Model file for the job. Use its own axes, mm. Face numbers are marked on the shaded views. A direction names the side the tool comes from. Coordinates: 2 decimals unless noted, no trailing zeros. Order: outer loops, then holes, each group sorted by start corner. A loop starts at its lowest first (then second) coordinate and runs counter-clockwise, first axis right, second up.
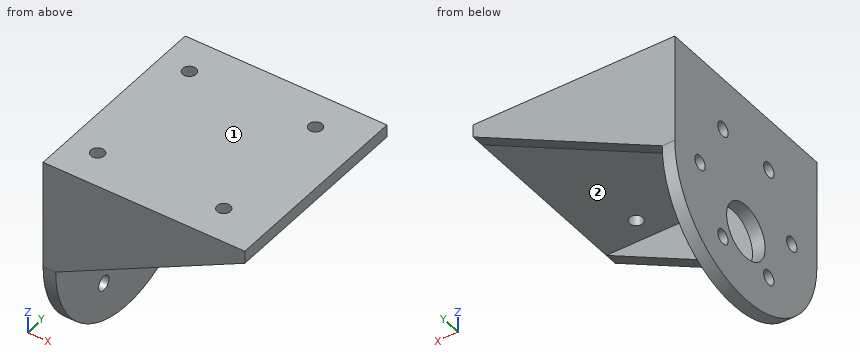
from build123d import *

# Parameters (mm, degrees)
SKETCH1_W           = 45
SKETCH1_H           = 48
SKETCH1_R           = 1.6
BOSS_EXTRUDE1_DEPTH = 3
BOSS_EXTRUDE2_DEPTH = 3
SKETCH4_R           = 6.5
SKETCH4_R_2         = 1.75
CUT_EXTRUDE1_DEPTH  = 10
BOSS_EXTRUDE3_DEPTH = 3
BOSS_EXTRUDE4_START = -48
BOSS_EXTRUDE4_DEPTH = 3


with BuildPart() as part:
    # Sketch1 → Boss-Extrude1 (new body)
    with BuildSketch(Plane.XY):
        with Locations((22.5, 24)):
            Rectangle(SKETCH1_W, SKETCH1_H)
        with Locations((4, 8.5)):
            Circle(SKETCH1_R, mode=Mode.SUBTRACT)
        with Locations((4, 39.5)):
            Circle(SKETCH1_R, mode=Mode.SUBTRACT)
        with Locations((34, 8.5)):
            Circle(SKETCH1_R, mode=Mode.SUBTRACT)
        with Locations((34, 39.5)):
            Circle(SKETCH1_R, mode=Mode.SUBTRACT)
    extrude(amount=BOSS_EXTRUDE1_DEPTH)

    # Sketch2 → Boss-Extrude2 (add)
    with BuildSketch(Plane.ZY):
        with BuildLine():
            Line((3, 48), (-23, 48))
            ThreePointArc((-23, 48), (-47, 24), (-23, 0))
            Line((-23, 0), (3, 0))
            Line((3, 0), (3, 48))
        make_face()
    extrude(amount=BOSS_EXTRUDE2_DEPTH)

    # Sketch4 → Cut-Extrude1 (cut)
    with BuildSketch(Plane.ZY.offset(3)):
        with Locations((-30, 24)):
            Circle(SKETCH4_R)
        with Locations((-23, 39.5)):
            Circle(SKETCH4_R_2)
        with Locations((-9.576606241, 31.75)):
            Circle(SKETCH4_R_2)
        with Locations((-9.576606241, 16.25)):
            Circle(SKETCH4_R_2)
        with Locations((-23, 8.5)):
            Circle(SKETCH4_R_2)
        with Locations((-36.423393759, 16.25)):
            Circle(SKETCH4_R_2)
        with Locations((-36.423393759, 31.75)):
            Circle(SKETCH4_R_2)
    extrude(amount=-CUT_EXTRUDE1_DEPTH, mode=Mode.SUBTRACT)

    # Sketch5 → Boss-Extrude3 (add)
    with BuildSketch(Plane(origin=(0, 48, 0), x_dir=(1, 0, 0), z_dir=(0, 1, 0))):
        Polygon((0, 23), (45, 0), (0, 0), align=None)
    extrude(amount=-BOSS_EXTRUDE3_DEPTH)

    # Sketch5<2> → Boss-Extrude4 (add)
    with BuildSketch(Plane(origin=(0, 48, 0), x_dir=(1, 0, 0), z_dir=(0, 1, 0)).offset(BOSS_EXTRUDE4_START)):
        Polygon((0, 23), (45, 0), (0, 0), align=None)
    extrude(amount=BOSS_EXTRUDE4_DEPTH)


solid = part.part
Q1. Cut at B-B, the plane y = 39.5. List the corners of the cut face in (x, z), plus the area to 3 significant figures.
Established:
outline: (-3, -41.32) - (0, -41.32) - (0, -24.75) - (-3, -24.75) - close; (-3, -21.25) - (0, -21.25) - (0, 0) - (2.4, 0) - (2.4, 3) - (-3, 3) - close; (5.6, 0) - (32.4, 0) - (32.4, 3) - (5.6, 3) - close; (35.6, 0) - (45, 0) - (45, 3) - (35.6, 3) - close
area: 238 mm2
Q2. Cut at C-C, the plane x = 4. List the corners of the cut face in (y, z), plus the area to 3 significant figures.
Established:
outline: (0, -20.96) - (3, -20.96) - (3, 0) - (6.9, 0) - (6.9, 3) - (0, 3) - close; (10.1, 0) - (37.9, 0) - (37.9, 3) - (10.1, 3) - close; (41.1, 0) - (45, 0) - (45, -20.96) - (48, -20.96) - (48, 3) - (41.1, 3) - close
area: 251 mm2
Q3. Drop flat-ended pins along their axis: P1, Ø2, axis at y = 16.25, z = -9.58, coming from the -X side; P2, Ø1.5, axis at y = 35.5, z = -19, coming from the +X side; P3, Ø3, axis at x = 4.5, y = 39.5, coming from the -Z side; P4, Ø18.5, axis at x = 16.5, z = -7, coming from the -Y side. Give the stop position or say it passes through.
Established:
P1: passes through
P2: stops at x = 0
P3: stops at z = 0
P4: stops at y = 0
Q4. Probe line 1 (X direction, y = 8, z = 2); line 2 (Z direction, x = -1, y = 16); line 3 (Y direction, x = 42, z = -1.5). List the from-to ranges inside material, lowest first.
Established:
line 1: x = -3 to 2.48, 5.52 to 32.48, 35.52 to 45
line 2: z = -45.63 to -38.16, -34.69 to -11.31, -7.84 to 3
line 3: y = 0 to 3, 45 to 48
Q5. Which spindle directions (+Z, -Z, +X, -X, +Y, -Y) get a long thin tool onto all of the face, cutting with end or side? Do the marked faces 1 and 2. Say none if no direction does.
Established:
face 1: +Z, +X, -X, +Y, -Y
face 2: -Z, +X
Q6. Cut at D-D, the plane z = -30. List the corners of the cut face in (x, y), plus the area to 3 significant figures.
Established:
outline: (-3, 1.04) - (0, 1.04) - (0, 17.5) - (-3, 17.5) - close; (-3, 30.5) - (0, 30.5) - (0, 46.96) - (-3, 46.96) - close
area: 98.7 mm2
Q7. Cut at A-A, the plane z = -9. List the corners of the cut face in (x, y).
Established:
outline: (-3, 0) - (27.39, 0) - (27.39, 3) - (0, 3) - (0, 14.6) - (-3, 14.6) - close; (-3, 17.9) - (0, 17.9) - (0, 30.1) - (-3, 30.1) - close; (-3, 33.4) - (0, 33.4) - (0, 45) - (27.39, 45) - (27.39, 48) - (-3, 48) - close
